Answer from the drawing. Dimensions are ordinates in mm from the lowest x, y and z of the part. A direction names the side the tool comes from. Round coordinates to 2 decimals unless told otherwise and drop trailing zeros. Order: outer loops, then holes, each group sorted by start corner. A loop starts at its lowest first (then second) coordinate and runs counter-clockwise, first axis right, second up.
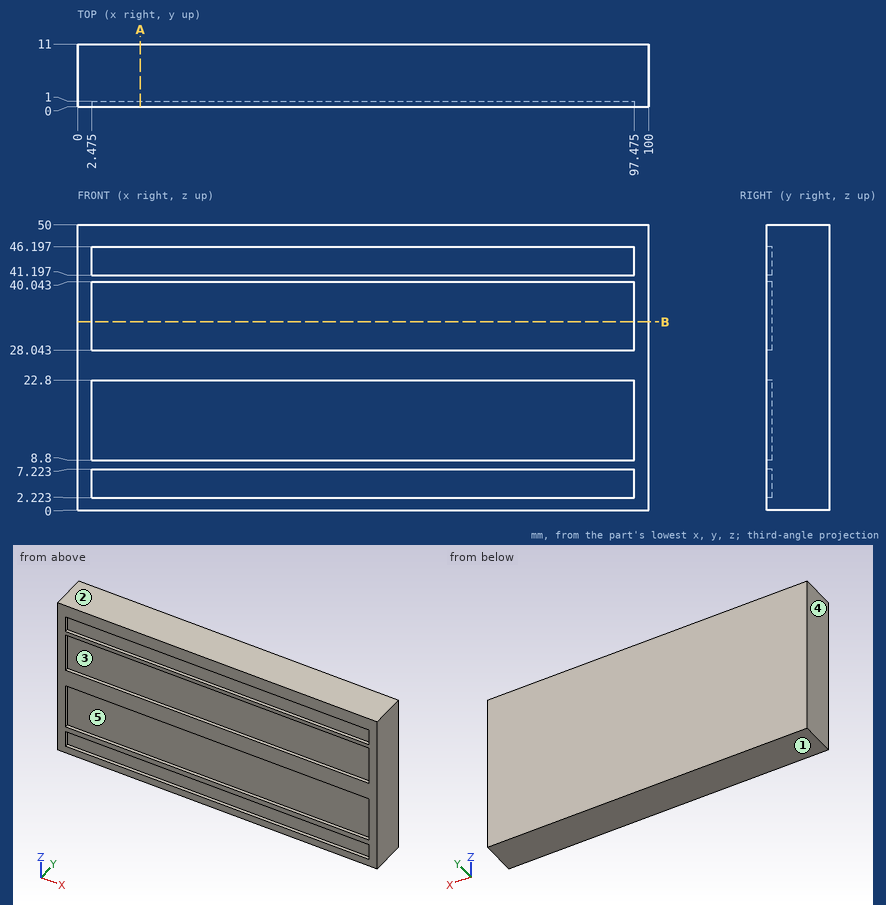
Q1. For the marked faces 4 and 5, determine the directions among +Z, -Z, +X, -X, +Y, -Y from which every point of the face is accessible in a straight line to the end or side of a thin tool.
Outcome:
face 4: +Z, -Z, -X, +Y, -Y
face 5: -Y
Q2. Flat-ended cylindrical pins translate along their axes: pin 1 (0.5 mm diameter, centred on y = 0.5, z = 31.5, fed in from -X); pin 2 (1.5 mm diameter, centred on x = 43.5, z = 5, fed in from -Y). Find the tip coordinate at first contact, or state that the pin passes through.
Outcome:
pin 1: stops at x = 0
pin 2: stops at y = 1
Q3. A cutting plane is placed at B-B, the plane z = 33. Give the vertices of the cut face in (x, y) (1 decimal), plus the area to 4 significant figures.
Outcome:
outline: (0, 0) - (2.5, 0) - (2.5, 1) - (97.5, 1) - (97.5, 0) - (100, 0) - (100, 11) - (0, 11) - close
area: 1,005 mm2
Q4. For a pull along Z with two mould halves and no side action, classify the marked faces 1, 2 and 3 as released by +Z, released by -Z, zero draft, split by the parting line, or undercut.
Outcome:
face 1: released by -Z
face 2: released by +Z
face 3: undercut
Q5. A cutting plane is placed at A-A, the plane x = 11. Give the vertices of the cut face in (y, z), plus the area to 3 significant figures.
Outcome:
outline: (0, 0) - (11, 0) - (11, 50) - (0, 50) - (0, 46.2) - (1, 46.2) - (1, 41.2) - (0, 41.2) - (0, 40.04) - (1, 40.04) - (1, 28.04) - (0, 28.04) - (0, 22.8) - (1, 22.8) - (1, 8.8) - (0, 8.8) - (0, 7.22) - (1, 7.22) - (1, 2.22) - (0, 2.22) - close
area: 514 mm2
Q6. A straight line is drawn through the part: probe 1 along Y at (x, z) = (20.5, 36). Find the intervals that lie inside material, in ascending order.
Outcome:
probe 1: y = 1 to 11
